```python
from build123d import *

# Parameters (mm, degrees)
F0_R          = 15
F1_DEPTH      = 100
F3_DEPTH      = 40
F5_R          = 4
F6_DEPTH      = 25
F6_DEPTH_BACK = 25


# Not quite as in the source:
# - a fillet or chamfer that OpenCascade refuses, or shapes differently, is made with other operations: its cross-section is extruded or revolved along the edge and cut away or added


with BuildPart() as f1:
    # F0 (on Top) → F1 (new body)
    with BuildSketch(Plane.XY):
        Circle(F0_R)
    extrude(amount=F1_DEPTH)

    # F2 (on face) → F3 (cut)
    with BuildSketch(Plane.XY.offset(100)):
        with BuildLine():
            Line((9.1818189363, 0), (11.1818189363, 0))
            ThreePointArc((11.1818189363, 0), (0.1818189363, 11), (-10.8181810637, 0))
            Line((-10.8181810637, 0), (-8.8181810637, 0))
            ThreePointArc((-8.8181810637, 0), (0.1818189363, 9), (9.1818189363, 0))
        make_face()
    extrude(amount=-F3_DEPTH, mode=Mode.SUBTRACT)

    # F4: fillet of radius 5 on 2 edges, made by hand

    # F4_s1 → F4_t2 (revolve, cut)
    with BuildSketch(Plane.XZ):
        with BuildLine():
            ThreePointArc((15, 95), (13.5355339059, 98.5355339059), (10, 100))
            Line((10, 100), (15, 100))
            Line((15, 100), (15, 95))
        make_face()
    revolve(axis=Axis((0, 0, 100), (0, 0, 1)), mode=Mode.SUBTRACT)

    # F4_s3 → F4_t4 (revolve, cut)
    with BuildSketch(Plane.XZ):
        with BuildLine():
            ThreePointArc((15, 5), (13.5355339059, 1.4644660941), (10, 0))
            Line((10, 0), (15, 0))
            Line((15, 0), (15, 5))
        make_face()
    revolve(axis=Axis((0, 0, 0), (0, 0, 1)), mode=Mode.SUBTRACT)

    # F5 (on Front) → F6 (cut, two sides)
    with BuildSketch(Plane.XZ) as f6_sk:
        with Locations((0, 20)):
            Circle(F5_R)
    extrude(amount=-F6_DEPTH, mode=Mode.SUBTRACT)
    extrude(f6_sk.sketch, amount=F6_DEPTH_BACK, mode=Mode.SUBTRACT)


solid = f1.part
```
Build history of the part. All positions in model axes, mm. A direction names the side the tool comes from. Give positions to 0.01 mm unless a question says otherwise; leave off trailing zeros. Loops run counter-clockwise (first coordinate to the right, second up) from the corner with the lowest first, then second, coordinate; pieces in that order, holes last.
Item 1: Slice it at B-B, the plane x = 0. List the corners of the cut face in (y, z).
Answers follow:
outline: (-15, 5) arc R5 ccw to (-10, 0) - (10, 0) arc R5 ccw to (15, 5) - (15, 16) - (-15, 16) - close; (-15, 24) - (15, 24) - (15, 95) arc R5 ccw to (11, 99.9) - (11, 60) - (9, 60) - (9, 100) - (-10, 100) arc R5 ccw to (-15, 95) - close
Item 2: Which spindle directions (+Z, -Z, +X, -X, +Y, -Y) get a long thin tool onto all of the face, cutting with end or side? Do faces 4 (the face through (10, 0, 80)), 5 (the face through (0, 0, 100)). Say none if no direction does.
Answers follow:
face 4: +Z
face 5: +Z, +X, -X, +Y, -Y
Item 3: Drill centre lines: line 1 (Z direction, x = 0, y = -9); line 2 (X direction, y = 8, z = 63); line 3 (X direction, y = 3, z = 20). Where is each one in solid material? Low to high.
Answers follow:
line 1: z = 0 to 16, 24 to 100
line 2: x = -12.69 to -7.37, -3.94 to 4.3, 7.73 to 12.69
line 3: x = -14.7 to -4, 4 to 14.7
Item 4: Flat gauge pins, fed straight in: pin 1 (2 mm diameter, centred on y = 3, z = 54.5, fed in from -X); pin 2 (1.5 mm diameter, centred on x = -8, z = 57.5, fed in from +Y); pin 3 (1.5 mm diameter, centred on x = -12, z = 55, fed in from -Y); pin 4 (2 mm diameter, centred on x = -11.5, y = -11.5, fed in from -Z). Where does each tip first touch, or does it go through?
Answers follow:
pin 1: stops at x = -14.87
pin 2: stops at y = 13.13
pin 3: stops at y = -9.92
pin 4: passes through
Item 5: Pull direction Y, two halves, no side cores. Call faces 1 (the face through (-0.7, 9.2, 60)), 2 (the face through (0, 0, 0)), 3 (the face through (14.307, 4.506, 49.37)): released by +Y, released by -Y, zero draft, split by the parting line, or undercut.
Answers follow:
face 1: undercut
face 2: zero draft
face 3: split by the parting line
Item 6: Slice it at A-A, the plane z = 62. List the corners of the cut face in (x, y), and give its area (3 significant figures).
Answers follow:
outline: circle Ø30 at (0, 0); hole (-10.82, 0) - (-8.82, 0) arc R9 cw to (9.18, 0) - (11.18, 0) arc R11 ccw to start
area: 644 mm2
Item 7: Slice it at C-C, the plane z = 20. List the corners of the cut face in (x, y), and give its area (3 significant figures).
Answers follow:
outline: (-4, -14.46) - (-4, 14.46) arc R15 ccw to start; (4, -14.46) arc R15 ccw to (4, 14.46) - close
area: 470 mm2
